from build123d import *

# Parameters (mm, degrees)
F0_W     = 2.5
F0_H     = 50
F1_DEPTH = 2
F2_DEPTH = 4
F3_DEPTH = 4
F4_DEPTH = 10


with BuildPart() as f1:
    # F0 (on Top) → F1 (new body)
    with BuildSketch(Plane.XY):
        with BuildLine():
            ThreePointArc((-32.5, -25), (-31.6213203436, -27.1213203436), (-29.5, -28))
            Line((-29.5, -28), (-29.0716141462, -28))
            Line((-29.0716141462, -28), (49.5, -28))
            ThreePointArc((49.5, -28), (51.6213203436, -27.1213203436), (52.5, -25))
            Line((52.5, -25), (50, -25))
            Line((50, -25), (50, 25))
            Line((50, 25), (52.5, 25))
            ThreePointArc((52.5, 25), (51.6213203436, 27.1213203436), (49.5, 28))
            Line((49.5, 28), (-29.5, 28))
            ThreePointArc((-29.5, 28), (-31.6213203436, 27.1213203436), (-32.5, 25))
            Line((-32.5, 25), (-32.5, -24.5))
            Line((-32.5, -24.5), (-32.5, -25))
        make_face()
        with BuildLine():
            ThreePointArc((-29, 22.125), (-30.6793786053, 26.1793786053), (-26.625, 24.5))
            Line((-26.625, 24.5), (26.625, 24.5))
            ThreePointArc((26.625, 24.5), (29, 26.875), (31.375, 24.5))
            ThreePointArc((31.375, 24.5), (30.6793786053, 22.8206213947), (29, 22.125))
            Line((29, 22.125), (29, -22.125))
            ThreePointArc((29, -22.125), (30.6793786053, -22.8206213947), (31.375, -24.5))
            ThreePointArc((31.375, -24.5), (29, -26.875), (26.625, -24.5))
            Line((26.625, -24.5), (-26.625, -24.5))
            ThreePointArc((-26.625, -24.5), (-30.6793786053, -26.1793786053), (-29, -22.125))
            Line((-29, -22.125), (-29, 22.125))
        make_face(mode=Mode.SUBTRACT)
        with BuildLine():
            Line((26.625, 24.5), (-26.625, 24.5))
            ThreePointArc((-26.625, 24.5), (-27.3206213947, 22.8206213947), (-29, 22.125))
            Line((-29, 22.125), (-29, -22.125))
            ThreePointArc((-29, -22.125), (-27.3206213947, -22.8206213947), (-26.625, -24.5))
            Line((-26.625, -24.5), (26.625, -24.5))
            ThreePointArc((26.625, -24.5), (27.3206213947, -22.8206213947), (29, -22.125))
            Line((29, -22.125), (29, 22.125))
            ThreePointArc((29, 22.125), (27.3206213947, 22.8206213947), (26.625, 24.5))
        make_face()
        with BuildLine():
            Line((-29, 23.125), (-29, 24.5))
            Line((-29, 24.5), (-27.625, 24.5))
            ThreePointArc((-27.625, 24.5), (-29.9722718241, 25.4722718241), (-29, 23.125))
        make_face()
        with BuildLine():
            ThreePointArc((-29, 23.125), (-29.9722718241, 25.4722718241), (-27.625, 24.5))
            Line((-27.625, 24.5), (-26.625, 24.5))
            ThreePointArc((-26.625, 24.5), (-30.6793786053, 26.1793786053), (-29, 22.125))
            Line((-29, 22.125), (-29, 23.125))
        make_face()
        with BuildLine():
            Line((-27.625, 24.5), (-29, 24.5))
            Line((-29, 24.5), (-29, 23.125))
            ThreePointArc((-29, 23.125), (-28.0277281759, 23.5277281759), (-27.625, 24.5))
        make_face()
        with BuildLine():
            Line((-26.625, 24.5), (-27.625, 24.5))
            ThreePointArc((-27.625, 24.5), (-28.0277281759, 23.5277281759), (-29, 23.125))
            Line((-29, 23.125), (-29, 22.125))
            ThreePointArc((-29, 22.125), (-27.3206213947, 22.8206213947), (-26.625, 24.5))
        make_face()
        with BuildLine():
            Line((-29, -24.5), (-29, -23.125))
            ThreePointArc((-29, -23.125), (-29.9722718241, -25.4722718241), (-27.625, -24.5))
            Line((-27.625, -24.5), (-29, -24.5))
        make_face()
        with BuildLine():
            Line((-29, -23.125), (-29, -22.125))
            ThreePointArc((-29, -22.125), (-30.6793786053, -26.1793786053), (-26.625, -24.5))
            Line((-26.625, -24.5), (-27.625, -24.5))
            ThreePointArc((-27.625, -24.5), (-29.9722718241, -25.4722718241), (-29, -23.125))
        make_face()
        with BuildLine():
            ThreePointArc((-27.625, -24.5), (-28.0277281759, -23.5277281759), (-29, -23.125))
            Line((-29, -23.125), (-29, -24.5))
            Line((-29, -24.5), (-27.625, -24.5))
        make_face()
        with BuildLine():
            ThreePointArc((-26.625, -24.5), (-27.3206213947, -22.8206213947), (-29, -22.125))
            Line((-29, -22.125), (-29, -23.125))
            ThreePointArc((-29, -23.125), (-28.0277281759, -23.5277281759), (-27.625, -24.5))
            Line((-27.625, -24.5), (-26.625, -24.5))
        make_face()
        with BuildLine():
            Line((29, -23.125), (29, -22.125))
            ThreePointArc((29, -22.125), (27.3206213947, -22.8206213947), (26.625, -24.5))
            Line((26.625, -24.5), (27.625, -24.5))
            ThreePointArc((27.625, -24.5), (28.0277281759, -23.5277281759), (29, -23.125))
        make_face()
        with BuildLine():
            Line((29, -24.5), (29, -23.125))
            ThreePointArc((29, -23.125), (28.0277281759, -23.5277281759), (27.625, -24.5))
            Line((27.625, -24.5), (29, -24.5))
        make_face()
        with BuildLine():
            ThreePointArc((31.375, -24.5), (30.6793786053, -22.8206213947), (29, -22.125))
            Line((29, -22.125), (29, -23.125))
            ThreePointArc((29, -23.125), (29.9722718241, -23.5277281759), (30.375, -24.5))
            ThreePointArc((30.375, -24.5), (29, -25.875), (27.625, -24.5))
            Line((27.625, -24.5), (26.625, -24.5))
            ThreePointArc((26.625, -24.5), (29, -26.875), (31.375, -24.5))
        make_face()
        with BuildLine():
            ThreePointArc((30.375, -24.5), (29.9722718241, -23.5277281759), (29, -23.125))
            Line((29, -23.125), (29, -24.5))
            Line((29, -24.5), (27.625, -24.5))
            ThreePointArc((27.625, -24.5), (29, -25.875), (30.375, -24.5))
        make_face()
        with BuildLine():
            ThreePointArc((31.375, 24.5), (29, 26.875), (26.625, 24.5))
            Line((26.625, 24.5), (27.625, 24.5))
            ThreePointArc((27.625, 24.5), (29, 25.875), (30.375, 24.5))
            ThreePointArc((30.375, 24.5), (29.9722718241, 23.5277281759), (29, 23.125))
            Line((29, 23.125), (29, 22.125))
            ThreePointArc((29, 22.125), (30.6793786053, 22.8206213947), (31.375, 24.5))
        make_face()
        with BuildLine():
            ThreePointArc((30.375, 24.5), (29, 25.875), (27.625, 24.5))
            Line((27.625, 24.5), (29, 24.5))
            Line((29, 24.5), (29, 23.125))
            ThreePointArc((29, 23.125), (29.9722718241, 23.5277281759), (30.375, 24.5))
        make_face()
        with BuildLine():
            Line((29, 24.5), (27.625, 24.5))
            ThreePointArc((27.625, 24.5), (28.0277281759, 23.5277281759), (29, 23.125))
            Line((29, 23.125), (29, 24.5))
        make_face()
        with BuildLine():
            Line((27.625, 24.5), (26.625, 24.5))
            ThreePointArc((26.625, 24.5), (27.3206213947, 22.8206213947), (29, 22.125))
            Line((29, 22.125), (29, 23.125))
            ThreePointArc((29, 23.125), (28.0277281759, 23.5277281759), (27.625, 24.5))
        make_face()
        with Locations((51.25, 0)):
            Rectangle(F0_W, F0_H)
    extrude(amount=F1_DEPTH)

    # F0 (on Top) → F2 (join)
    with BuildSketch(Plane.XY):
        with Locations((51.25, 0)):
            Rectangle(F0_W, F0_H)
    extrude(amount=F2_DEPTH)

    # F0 (on Top) → F3 (join)
    with BuildSketch(Plane.XY):
        with BuildLine():
            Line((-29, -23.125), (-29, -22.125))
            ThreePointArc((-29, -22.125), (-30.6793786053, -26.1793786053), (-26.625, -24.5))
            Line((-26.625, -24.5), (-27.625, -24.5))
            ThreePointArc((-27.625, -24.5), (-29.9722718241, -25.4722718241), (-29, -23.125))
        make_face()
        with BuildLine():
            ThreePointArc((-26.625, -24.5), (-27.3206213947, -22.8206213947), (-29, -22.125))
            Line((-29, -22.125), (-29, -23.125))
            ThreePointArc((-29, -23.125), (-28.0277281759, -23.5277281759), (-27.625, -24.5))
            Line((-27.625, -24.5), (-26.625, -24.5))
        make_face()
        with BuildLine():
            Line((29, -23.125), (29, -22.125))
            ThreePointArc((29, -22.125), (27.3206213947, -22.8206213947), (26.625, -24.5))
            Line((26.625, -24.5), (27.625, -24.5))
            ThreePointArc((27.625, -24.5), (28.0277281759, -23.5277281759), (29, -23.125))
        make_face()
        with BuildLine():
            ThreePointArc((31.375, -24.5), (30.6793786053, -22.8206213947), (29, -22.125))
            Line((29, -22.125), (29, -23.125))
            ThreePointArc((29, -23.125), (29.9722718241, -23.5277281759), (30.375, -24.5))
            ThreePointArc((30.375, -24.5), (29, -25.875), (27.625, -24.5))
            Line((27.625, -24.5), (26.625, -24.5))
            ThreePointArc((26.625, -24.5), (29, -26.875), (31.375, -24.5))
        make_face()
        with BuildLine():
            ThreePointArc((31.375, 24.5), (29, 26.875), (26.625, 24.5))
            Line((26.625, 24.5), (27.625, 24.5))
            ThreePointArc((27.625, 24.5), (29, 25.875), (30.375, 24.5))
            ThreePointArc((30.375, 24.5), (29.9722718241, 23.5277281759), (29, 23.125))
            Line((29, 23.125), (29, 22.125))
            ThreePointArc((29, 22.125), (30.6793786053, 22.8206213947), (31.375, 24.5))
        make_face()
        with BuildLine():
            Line((27.625, 24.5), (26.625, 24.5))
            ThreePointArc((26.625, 24.5), (27.3206213947, 22.8206213947), (29, 22.125))
            Line((29, 22.125), (29, 23.125))
            ThreePointArc((29, 23.125), (28.0277281759, 23.5277281759), (27.625, 24.5))
        make_face()
        with BuildLine():
            ThreePointArc((-29, 23.125), (-29.9722718241, 25.4722718241), (-27.625, 24.5))
            Line((-27.625, 24.5), (-26.625, 24.5))
            ThreePointArc((-26.625, 24.5), (-30.6793786053, 26.1793786053), (-29, 22.125))
            Line((-29, 22.125), (-29, 23.125))
        make_face()
        with BuildLine():
            Line((-26.625, 24.5), (-27.625, 24.5))
            ThreePointArc((-27.625, 24.5), (-28.0277281759, 23.5277281759), (-29, 23.125))
            Line((-29, 23.125), (-29, 22.125))
            ThreePointArc((-29, 22.125), (-27.3206213947, 22.8206213947), (-26.625, 24.5))
        make_face()
    extrude(amount=F3_DEPTH)

    # F0 (on Top) → F4 (join)
    with BuildSketch(Plane.XY):
        with BuildLine():
            ThreePointArc((30.375, -24.5), (29.9722718241, -23.5277281759), (29, -23.125))
            Line((29, -23.125), (29, -24.5))
            Line((29, -24.5), (27.625, -24.5))
            ThreePointArc((27.625, -24.5), (29, -25.875), (30.375, -24.5))
        make_face()
        with BuildLine():
            Line((29, -24.5), (29, -23.125))
            ThreePointArc((29, -23.125), (28.0277281759, -23.5277281759), (27.625, -24.5))
            Line((27.625, -24.5), (29, -24.5))
        make_face()
        with BuildLine():
            Line((-29, -24.5), (-29, -23.125))
            ThreePointArc((-29, -23.125), (-29.9722718241, -25.4722718241), (-27.625, -24.5))
            Line((-27.625, -24.5), (-29, -24.5))
        make_face()
        with BuildLine():
            ThreePointArc((-27.625, -24.5), (-28.0277281759, -23.5277281759), (-29, -23.125))
            Line((-29, -23.125), (-29, -24.5))
            Line((-29, -24.5), (-27.625, -24.5))
        make_face()
        with BuildLine():
            Line((-29, 23.125), (-29, 24.5))
            Line((-29, 24.5), (-27.625, 24.5))
            ThreePointArc((-27.625, 24.5), (-29.9722718241, 25.4722718241), (-29, 23.125))
        make_face()
        with BuildLine():
            Line((-27.625, 24.5), (-29, 24.5))
            Line((-29, 24.5), (-29, 23.125))
            ThreePointArc((-29, 23.125), (-28.0277281759, 23.5277281759), (-27.625, 24.5))
        make_face()
        with BuildLine():
            ThreePointArc((30.375, 24.5), (29, 25.875), (27.625, 24.5))
            Line((27.625, 24.5), (29, 24.5))
            Line((29, 24.5), (29, 23.125))
            ThreePointArc((29, 23.125), (29.9722718241, 23.5277281759), (30.375, 24.5))
        make_face()
        with BuildLine():
            Line((29, 24.5), (27.625, 24.5))
            ThreePointArc((27.625, 24.5), (28.0277281759, 23.5277281759), (29, 23.125))
            Line((29, 23.125), (29, 24.5))
        make_face()
    extrude(amount=F4_DEPTH)


solid = f1.part
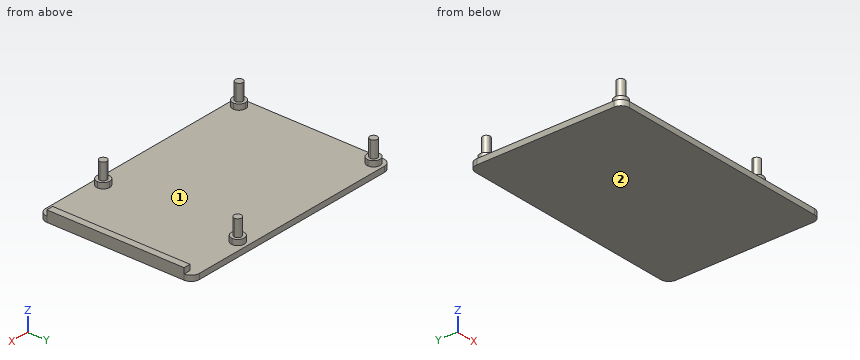
Build history of the part. All positions in model axes, mm. Face numbers are marked on the shaded views. A direction names the side the tool comes from. Round coordinates to 2 decimals unless told otherwise and drop trailing zeros. Write each loop counter-clockwise with the first axis right and the second up, starting at its lowest first coordinate (ties: lowest second). Pieces come first, ordered by that corner, then holes. Notation, with made-up numbers: M -27,3 L -9,3 A13 ccw -9,19 Z; hole C -26.5,72 d10. An arc over 180 degrees is marked long. Answer as a JSON object with one key per item and string values. Group by question number.
(1) Cut at A-A (z = 5). Give the cut face in (x, y) (3 decimals).
(2) Which spindle directions (+Z, -Z, +X, -X, +Y, -Y) get a long thin tool onto all of the face, cutting with end or side? Do the marked faces 1 and 2. Say none if no direction does.
(3) Cut at B-B (y = 9.5). Give the cut face in (x, z).
(4) Cut at C-C (x = 19). Give the cut face in (y, z), and give its area (3 significant figures).
(5) Flat gauge pins, fed straight in: pin 1 (1.6 mm diameter, centred on x = 51.5, z = 2.5, fed in from +Y); pin 2 (8 mm diameter, centred on x = 6.5, y = 13, fed in from +Z); pin 3 (1.2 mm diameter, centred on x = 51.5, y = 9.5, fed in from +Z). Where does each tip first touch, or does it go through?
(6) Drill centre lines: L1, parallel to Z at x = -4.5, y = 22.5; L2, parallel to X at y = -6.5, z = 3.75; L3, parallel to X at y = 24, z = 5. Where is each one in solid material? Low to high.
Responses:
{
 "1": {"outline": "C -29,-24.5 d2.75; C -29,24.5 d2.75; C 29,-24.5 d2.75; C 29,24.5 d2.75"},
 "2": {"face 1": "+Z", "face 2": "-Z, +X, -X, +Y, -Y"},
 "3": {"outline": "M -32.5,0 L 52.5,0 L 52.5,4 L 50,4 L 50,2 L -32.5,2 Z"},
 "4": {"outline": "M -28,0 L 28,0 L 28,2 L -28,2 Z", "area": "112 mm2"},
 "5": {"pin 1": "stops at y = 27.67", "pin 2": "stops at z = 2", "pin 3": "stops at z = 4"},
 "6": {"L1": "z = 0 to 2", "L2": "x = 50 to 52.5", "L3": "x = -30.28 to -27.72, 27.72 to 30.28"}
}
